The listing builds one solid part. Answer for the finished solid, in the listing's coordinates (mm). Face numbers are marked on the shaded views. Round coordinates to 2 decimals unless told otherwise and drop trailing zeros. Write each loop counter-clockwise with the first axis right and the second up, starting at its lowest first coordinate (ties: lowest second). Pieces come first, ordered by that corner, then holes. Notation, with made-up numbers: M -11.75,81 L 47.25,81 A31 cw 47.25,114 Z; hole C 73.25,-22.75 d9. An arc over 180 degrees is marked long. Write each question's results on one line, items separated by ' | '.
Autodesk Inventor part; units mm, degrees
ref_plane "YZ Plane" through (0, 0, 0) normal (1, 0, 0) x (0, 1, 0)
ref_plane "XZ Plane" through (0, 0, 0) normal (0, 1, 0) x (-1, 0, 0)
ref_plane "XY Plane" through (0, 0, 0) normal (0, 0, 1) x (1, 0, 0)
sketch "Sketch1" plane through (0, 0, 0) normal (0, 1, 0) x (-1, 0, 0)
  circle A0 centre (0, 0) radius 14.2875
  line L0 (0, 25.4) -> (0, -25.4) construction
  circle A1 centre (0, 0) radius 18.1864 construction
  circle A2 centre (0, 25.4) radius 4.7625 construction
  circle A3 centre (0, -25.4) radius 4.7625 construction
  circle A4 centre (0, 0) radius 20.6375 construction
  line L1 (16.1101, 12.8984) -> (3.7177, 28.3766)
  line L2 (16.1101, -12.8984) -> (3.7177, -28.3766)
  line L3 (-3.7177, -28.3766) -> (-16.1101, -12.8984)
  line L4 (-16.1101, 12.8984) -> (-3.7177, 28.3766)
  arc A5 (3.7177, 28.3766) -> (-3.7177, 28.3766) centre (0, 25.4) ccw
  arc A6 (-16.1101, 12.8984) -> (-16.1101, -12.8984) centre (0, 0) ccw
  arc A7 (16.1101, -12.8984) -> (16.1101, 12.8984) centre (0, 0) ccw
  arc A8 (-3.7177, -28.3766) -> (3.7177, -28.3766) centre (0, -25.4) ccw
  point P0 (-3.7177, 28.3766)
  point P1 (3.7177, -28.3766)
  dimension "d0" = 28.575
  dimension "d1" = 50.8
  dimension "d2" = 36.3728
  dimension "d3" = 9.525
  dimension "d4" = 9.525
  dimension "d5" = 6.35
extrude "Extrusion1" add sketch "Sketch1" along normal blind 6.35
hole "Hole1" at (0, 0, 25.4) at (0, 0, -25.4) direction (0, 1, 0) diameter 5.1054 end through all
properties part number "EL2-CGB-005" material "Aluminum 6061"
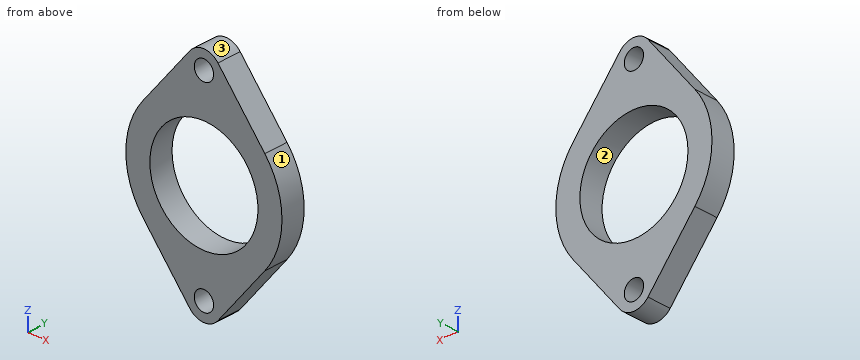
1) Each of these flat-tipped pins is pushed along its axis until it touches: pin 1 (4 mm diameter, centred on x = 15, z = 7, fed in from -Y); pin 2 (1 mm diameter, centred on y = 5.5, z = 1.5, fed in from +X); pin 3 (1 mm diameter, centred on y = 3, z = 15.5, fed in from +X); pin 4 (3 mm diameter, centred on y = 3.5, z = 17, fed in from +X). Where does it stop, or does it pass through?
Return value:
pin 1: y = 0 | pin 2: x = 20.61 | pin 3: x = 14.43 | pin 4: x = 14.03
2) The mould has two halves that part along Z. Classify the marked faces 1, 2 and 3: +Z half, -Z half, draft (parallel to the pull), parting line (faces both ways), or undercut.
Return value:
face 1: parting line | face 2: undercut | face 3: +Z half
3) Find the intervals of material crossed by line 1 (Z direction, x = 1, y = 6); line 2 (Z direction, x = -2, y = 5.75); line 3 (X direction, y = 2, z = -25.4), in increasing order.
Return value:
line 1: -30.06 to -27.75, -23.05 to -14.25, 14.25 to 23.05, 27.75 to 30.06 | line 2: -29.72 to -26.99, -23.81 to -14.15, 14.15 to 23.81, 26.99 to 29.72 | line 3: -6.1 to -2.55, 2.55 to 6.1
4) Section C-C (x = 0) is taken. Determine the outline of the cut face in (y, z), then the cut area to 3 significant figures.
Return value:
outline: M 0,-30.16 L 6.35,-30.16 L 6.35,-27.95 L 0,-27.95 Z; M 0,-22.85 L 6.35,-22.85 L 6.35,-14.29 L 0,-14.29 Z; M 0,14.29 L 6.35,14.29 L 6.35,22.85 L 0,22.85 Z; M 0,27.95 L 6.35,27.95 L 6.35,30.16 L 0,30.16 Z | area: 137 mm²
5) Section B-B (y = 1) is taken. Determine the outline of the cut face in (x, z) (1 decimal), then the cut area to 3 significant figures.
Return value:
outline: M -16.1,-12.9 L -3.7,-28.4 A4.8 ccw 3.7,-28.4 L 16.1,-12.9 A20.6 ccw 16.1,12.9 L 3.7,28.4 A4.8 ccw -3.7,28.4 L -16.1,12.9 A20.6 ccw Z; hole C 0,0 d28.6; hole C 0,-25.4 d5.1; hole C 0,25.4 d5.1 | area: 941 mm²
6) Section A-A (z = 0) is taken. Determine the outline of the cut face in (x, y).
Return value:
outline: M -20.64,0 L -14.29,0 L -14.29,6.35 L -20.64,6.35 Z; M 14.29,0 L 20.64,0 L 20.64,6.35 L 14.29,6.35 Z
7) Section D-D (x = 8) is taken. Determine the outline of the cut face in (y, z).
Return value:
outline: M 0,-23.03 L 6.35,-23.03 L 6.35,-11.84 L 0,-11.84 Z; M 0,11.84 L 6.35,11.84 L 6.35,23.03 L 0,23.03 Z
